```python
from build123d import *

# Parameters (mm, degrees)
SKETCH001_W  = 1.15
SKETCH001_H  = 1.85
POCKET_DEPTH = 5


with BuildPart() as part:
    # Sketch → Revolution (revolve)
    with BuildSketch(Plane.XZ):
        with BuildLine():
            ThreePointArc((0, 6), (1.321655, 6.210666), (2.512322, 6.821784))
            ThreePointArc((7.076375, 0), (6.107951, 4.289746), (2.512322, 6.821784))
            Line((7.076375, 0), (6.440959, 0))
            ThreePointArc((6.440959, 0), (5.315373, 2.832423), (2.5, 4))
            Line((2.5, 0), (2.5, 4))
            Line((0, 0), (2.5, 0))
            Line((0, 0), (0, 6))
        make_face()
    revolve(axis=Axis((0, 0, 0), (0, 0, 1)))

    # Sketch001 (on Face6 of Revolution) → Pocket (cut)
    with BuildSketch(Plane(origin=(0, 0, 0), x_dir=(1, 0, 0), z_dir=(0, 0, -1))):
        Rectangle(SKETCH001_W, SKETCH001_H)
    extrude(amount=-POCKET_DEPTH, mode=Mode.SUBTRACT)


solid = part.part
```
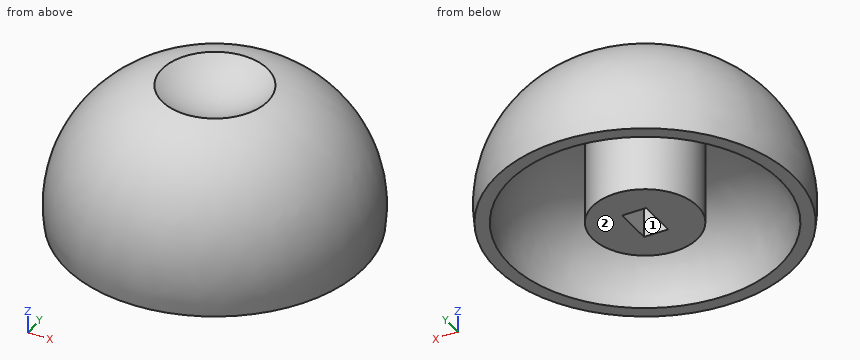
Geometry: final body of the model. Coordinates: model frame, mm. Face numbers are marked on the shaded views. Round coordinates to 2 decimals unless told otherwise and drop trailing zeros. Return JSON: item names as keys, results as strings.
Q1. First-contact query: pin 1 Ø2 at (x, z) = (4.5, 3) entering from -Y; pin 2 Ø1.3 at (x, y) = (-0.5, -0.5) entering from -Z; pin 3 Ø1 at (y, z) = (-5.5, 3) entering from +X; pin 4 Ø0.6 at (x, z) = (0, 2.5) entering from -Y. Flat tips, straight axial feed; report the tip coordinate or a pass-through.
From the geometry:
{"pin 1": "y = -5.9", "pin 2": "z = 0", "pin 3": "x = 4.61", "pin 4": "y = -7"}
Q2. Section A-A on z = 1.5. Give the number of separate pieces and of enclosed holes in the cut face, and give its area (3 significant figures).
From the geometry:
{"separate pieces": "2", "enclosed holes": "2", "area": "56.5 mm2"}
Q3. Ray query, line 1 (X direction, y = 0.5, z = 2.75) (3 decimals); line 2 (X direction, y = 0.5, z = 1.25) (3 decimals); line 3 (X direction, y = -2.25, z = 0.75). Return the intervals inside material, ascending.
From the geometry:
{"line 1": "-6.832 to -5.371, -2.449 to -0.575, 0.575 to 2.449, 5.371 to 6.832", "line 2": "-7.113 to -6.244, -2.449 to -0.575, 0.575 to 2.449, 6.244 to 7.113", "line 3": "-6.78 to -5.98, -1.09 to 1.09, 5.98 to 6.78"}
Q4. Mould query, pull axis Y, two halves, no side actions, for the marked faces 1 and 2. Classes: +Y half, -Y half, draft (parallel to the pull), parting line (faces both ways), or undercut.
From the geometry:
{"face 1": "undercut", "face 2": "draft"}
